Here's how the part is built. I have some questions about the finished solid (model axes, mm). Round coordinates to 2 decimals unless told otherwise and drop trailing zeros. Write each loop counter-clockwise with the first axis right and the second up, starting at its lowest first coordinate (ties: lowest second). Pieces come first, ordered by that corner, then holes. Notation, with made-up numbers: (77.25, 3.5) - (89.25, 3.5) arc R19 cw to (89.25, 8.5) - close; hole circle Ø11 at (28, 72.5). An arc over 180 degrees is marked (long way). Write item = value, one per line. Start each with the question number.
Item 1: For P1, Ø8, axis at x = 29, y = 148, coming from the -Z side; P2, Ø5, axis at y = 171.5, z = -4.5, coming from the -X side, each with a flat end and sliding along its axis, tell me the tip position at first contact or that it passes through.
Item 2: Thinking about a two-plate mould opening in Y: for faces 1 (the face through (68, 204, 0)), 2 (the face through (9, 435, 3)), 3 (the face through (55.3, -6.834, -3.042)), which applies, pulls with the +Y half, pulls with the -Y half, needs draft (parallel to the pull), parting line crosses it, or undercut?
Item 3: If we section it at A-A (y = 286): Please give me the cut outline in (x, z), and give its area (3 significant figures).
Item 4: If we section it at C-C (x = -37): Please give me the cut outline in (y, z), and give its area (3 significant figures).
Item 5: If we section it at B-B (z = -2.5): Please give me the cut outline in (x, y), and give its area (3 significant figures).
Item 6: If I drill on line 1 along Z through (x, y) = (9, 26); line 2 along Y through (x, z) = (-15, -0.5); line 3 along X through (y, z) = (245.5, -5.25), over which ranges is the centre line in solid material (lowest first)? Write a range as [from, to].
```python
from build123d import *

# Parameters (mm, degrees)
BOSS_EXTRUDE1_DEPTH = 6
SKETCH2_W           = 116
SKETCH2_H           = 455
BOSS_EXTRUDE2_DEPTH = 6
SKETCH3_R           = 10
CUT_EXTRUDE1_DEPTH  = 6


with BuildPart() as part:
    # Sketch1 → Boss-Extrude1 (new body)
    with BuildSketch(Plane.XY):
        Polygon((68, 435), (48, 435), (48, 0), (-48, 0), (-48, -20), (68, -20), align=None)
    extrude(amount=-BOSS_EXTRUDE1_DEPTH)

    # Sketch2 → Boss-Extrude2 (add)
    with BuildSketch(Plane.XY):
        with Locations((10, 207.5)):
            Rectangle(SKETCH2_W, SKETCH2_H)
    extrude(amount=BOSS_EXTRUDE2_DEPTH)

    # Sketch3 → Cut-Extrude1 (cut)
    with BuildSketch(Plane(origin=(0, 0, -6), x_dir=(-1, 0, 0), z_dir=(0, 0, -1))):
        with Locations((-48, 0)):
            Circle(SKETCH3_R)
    extrude(amount=-CUT_EXTRUDE1_DEPTH, mode=Mode.SUBTRACT)


solid = part.part
```
Reply:
q1.P1 = 0
q1.P2 = 48
q2.face_1 = needs draft
q2.face_2 = pulls with the +Y half
q2.face_3 = undercut
q3.outline = (-48, 0) - (48, 0) - (48, -6) - (68, -6) - (68, 6) - (-48, 6) - close
q3.area = 816 mm2
q4.outline = (-20, -6) - (0, -6) - (0, 0) - (435, 0) - (435, 6) - (-20, 6) - close
q4.area = 2,850 mm2
q5.outline = (-48, -20) - (68, -20) - (68, 435) - (48, 435) - (48, 10) arc R10 cw (long way) to (38, 0) - (-48, 0) - close
q5.area = 10,800 mm2
q6.line_1 = [0, 6]
q6.line_2 = [-20, 0]
q6.line_3 = [48, 68]
